Autodesk Inventor part; units mm, degrees
ref_plane "Start plane" through (0, 0, 0) normal (0, 0, 1) x (1, 0, 0)
ref_plane "End plane" through (0, 0, 980) normal (0, 0, 1) x (1, 0, 0)
ref_plane "Work Plane4" through (12, -900, 1020) normal (0, 0, 1) x (1, 0, 0)
ref_plane "Start plane" through (0, 0, 0) normal (0, 0, 1) x (1, 0, 0)
ref_plane "End plane" through (0, 0, 980) normal (0, 0, 1) x (1, 0, 0)
sketch "Sketch" plane through (0, 0, 0) normal (0, 0, 1) x (1, 0, 0)
  line L0 (-20, -12) -> (-20, 12)
  line L1 (-12, 20) -> (12, 20)
  line L2 (20, 12) -> (20, -12)
  line L3 (12, -20) -> (-12, -20)
  arc A0 (-20, -12) -> (-12, -20) centre (-12, -12) ccw
  arc A1 (-12, 20) -> (-20, 12) centre (-12, 12) ccw
  arc A2 (20, 12) -> (12, 20) centre (12, 12) ccw
  arc A3 (12, -20) -> (20, -12) centre (12, -12) ccw
  arc A4 (-12, 16) -> (-16, 12) centre (-12, 12) ccw
  line L4 (-12, 16) -> (12, 16)
  arc A5 (16, 12) -> (12, 16) centre (12, 12) ccw
  line L5 (16, 12) -> (16, -12)
  arc A6 (12, -16) -> (16, -12) centre (12, -12) ccw
  line L6 (12, -16) -> (-12, -16)
  arc A7 (-16, -12) -> (-12, -16) centre (-12, -12) ccw
  line L7 (-16, -12) -> (-16, 12)
  line L8 (0, 30.3196) -> (0, -30.3196) construction
  line L9 (-30.3196, 0) -> (30.3196, 0) construction
  dimension "d7" = 8
  dimension "d10" = 40
  dimension "d11" = 40
  dimension "d12" = 4
  dimension "d15" = 20
  dimension "d16" = 20
extrude "Body" add sketch "Sketch" along normal up to surface (980 mm away) from surface at 0
sketch "Sketch3" plane through (0, 0, 0) normal (0, 0, 1) x (1, 0, 0)
  line L0 (0, 0) -> (10, 0)
ref_plane "Work Plane3" through (0, 0, 0) normal (0, -1, 0) x (1, 0, 0)
sketch "Sketch4" plane through (0, 0, 0) normal (0, -1, 0) x (1, 0, 0)
  line L0 (-2, 0) -> (12, 0)
  line L1 (-2, 980) -> (12, 980)
  dimension "d18" = 980
ref_plane "Work Plane4" through (12, -900, 1020) normal (0, 0, 1) x (1, 0, 0)
split "Split1" plane through (12, -900, 1020) removes the side toward (0, 0, 1)
ref_plane "Work Plane5" through (-12, -900, 980) normal (0, 0, 1) x (1, 0, 0)
split "Split2" plane through (-12, -900, 980) removes the side toward (0, 0, 1)
equation "\"d7\" = G_IR"
equation "\"d10\" = G_H"
equation "\"d11\" = G_W"
equation "\"d12\" = G_T"
equation "\"d15\" = 0.5 * d10"
equation "\"d16\" = 0.5 * d11"
equation "\"d3\" = G_L"
equation "\"G_W\" = 40"
equation "\"G_H\" = 40"
equation "\"G_T\" = 4"
equation "\"G_IR\" = 8"
equation "\"G_L\" = d18"
equation "\"G_OFFSET_START\" = 0"
equation "\"G_OFFSET_END\" = -20"
equation "\"d14\" = G_OFFSET_END + B_L"
properties part number "DIN EN 10219-2 - 40 x 40 x 4  - 980" material "Steel, Mild"
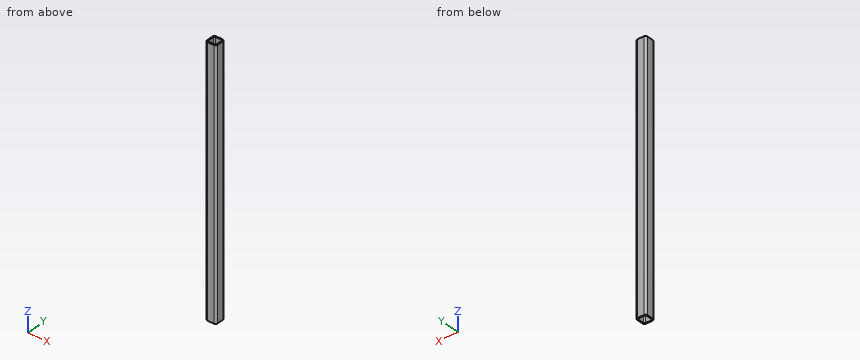
Source: CAD feature listing. Evaluate the final solid. Frame: model axes, mm. Give positions to 0.01 mm unless a question says otherwise; leave off trailing zeros. Write each loop counter-clockwise with the first axis right and the second up, starting at its lowest first coordinate (ties: lowest second). Pieces come first, ordered by that corner, then holes. Notation, with made-up numbers: (43, 23) - (52, 23) arc R24 cw to (52, 45) - close; hole circle Ø5 at (1, 20.25). An arc over 180 degrees is marked (long way). Write item = value, one per line. Start each with the question number.
Q1. Material intervals for probe 1 along X at (y, z) = (-7, 647); probe 2 along X at (y, z) = (13, 506.5), sorted ascending.
Q2. Cut plane A-A, the plane y = 6. Return loops of the section in (x, z), then the cut area to 3 significant figures.
Q3. Pin query (flat end, axial travel): pin 1 Ø1.5 at (x, y) = (-15, -11) entering from -Z. Return the tip coordinate at first contact, or that it passes through.
Q4. Cut plane B-B, the plane z = 221.5. Return loops of the section in (x, y), then the cut area to 3 significant figures.
Computed values:
q1.probe_1 = -20 to -16, 16 to 20
q1.probe_2 = -19.94 to -15.87, 15.87 to 19.94
q2.outline = (-20, 0) - (-16, 0) - (-16, 980) - (-20, 980) - close; (16, 0) - (20, 0) - (20, 980) - (16, 980) - close
q2.area = 7,840 mm²
q3.pin_1 = through
q4.outline = (-20, -12) arc R8 ccw to (-12, -20) - (12, -20) arc R8 ccw to (20, -12) - (20, 12) arc R8 ccw to (12, 20) - (-12, 20) arc R8 ccw to (-20, 12) - close; hole (-16, -12) arc R4 ccw to (-12, -16) - (12, -16) arc R4 ccw to (16, -12) - (16, 12) arc R4 ccw to (12, 16) - (-12, 16) arc R4 ccw to (-16, 12) - close
q4.area = 535 mm²
